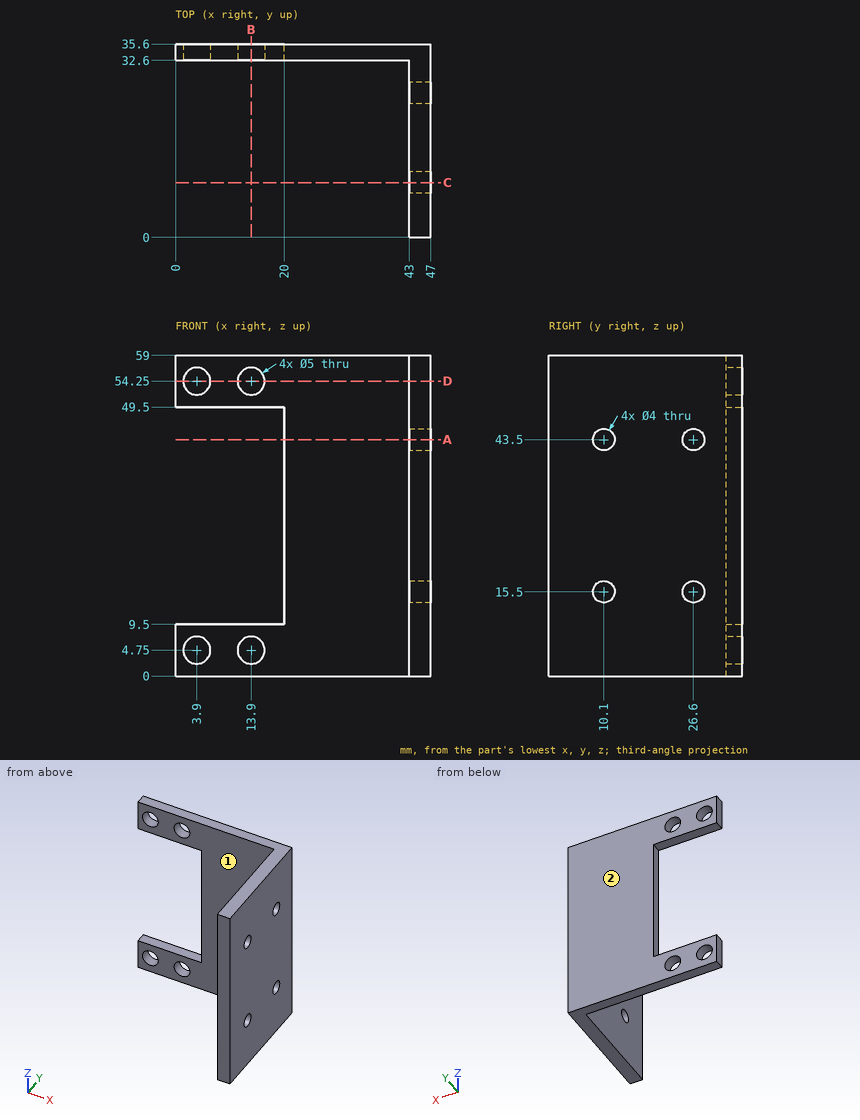
Source: three-view drawing plus pictorial views. Frame: mm from the lowest corner of the part. A direction names the side the tool comes from. Give positions to 0.01 mm unless a question says otherwise; leave off trailing zeros. Write each loop counter-clockwise with the first axis right and the second up, starting at its lowest first coordinate (ties: lowest second). Pieces come first, ordered by that corner, then holes. Notation, with made-up numbers: M -5,31 L 50,31 A17 ccw 50,61 Z; hole C -23.75,13 d9. An arc over 180 degrees is marked long. Use one line per item in the form item = value.
1. Cut plane A-A on z = 43.5. Return loops of the section in (x, y).
Outcome:
outline = M 20,32.6 L 43,32.6 L 43,28.6 L 47,28.6 L 47,35.6 L 20,35.6 Z; M 43,0 L 47,0 L 47,8.1 L 43,8.1 Z; M 43,12.1 L 47,12.1 L 47,24.6 L 43,24.6 Z
2. Ray query, L1, parallel to X at y = 34.4, z = 4.75; L2, parallel to Y at x = 44, z = 43.5; L3, parallel to Z at x = 13, y = 34. Return the intervals inside material, ascending.
Outcome:
L1 = 0 to 1.4, 6.4 to 11.4, 16.4 to 47
L2 = 0 to 8.1, 12.1 to 24.6, 28.6 to 35.6
L3 = 0 to 2.42, 7.08 to 9.5, 49.5 to 51.92, 56.58 to 59
3. Cut plane C-C on y = 10.1. Return loops of the section in (x, z).
Outcome:
outline = M 43,0 L 47,0 L 47,13.5 L 43,13.5 Z; M 43,17.5 L 47,17.5 L 47,41.5 L 43,41.5 Z; M 43,45.5 L 47,45.5 L 47,59 L 43,59 Z
4. Reachability of the marked faces 1 and 2 from +Z, -Z, +X, -X, +Y, -Y: full face, straight path, thin tool, end or side. Return the list, or none.
Outcome:
face_1 = +Z, -Z, -X, -Y
face_2 = +Z, -Z, +X, -X, +Y
5. Cut plane D-D on z = 54.25. Return loops of the section in (x, y), and give its area (3 significant figures).
Outcome:
outline = M 0,32.6 L 1.4,32.6 L 1.4,35.6 L 0,35.6 Z; M 6.4,32.6 L 11.4,32.6 L 11.4,35.6 L 6.4,35.6 Z; M 16.4,32.6 L 43,32.6 L 43,0 L 47,0 L 47,35.6 L 16.4,35.6 Z
area = 241 mm²
6. Cut plane B-B on x = 13.9. Return loops of the section in (y, z), and give its area (3 significant figures).
Outcome:
outline = M 32.6,0 L 35.6,0 L 35.6,2.25 L 32.6,2.25 Z; M 32.6,7.25 L 35.6,7.25 L 35.6,9.5 L 32.6,9.5 Z; M 32.6,49.5 L 35.6,49.5 L 35.6,51.75 L 32.6,51.75 Z; M 32.6,56.75 L 35.6,56.75 L 35.6,59 L 32.6,59 Z
area = 27.0 mm²
7. First-contact query: P1, Ø16.5, axis at y = 21, z = 38, coming from the -X side; P2, Ø3, axis at x = 20, z = 41.5, coming from the -Y side; P3, Ø2.5, axis at x = 14, y = 35, coming from the -Z side; P4, Ø3.5, axis at y = 34.5, z = 24.5, coming from the -X side. Flat tips, straight axial feed; report the tip coordinate or a pass-through.
Outcome:
P1 = 43
P2 = 32.6
P3 = 0
P4 = 20
